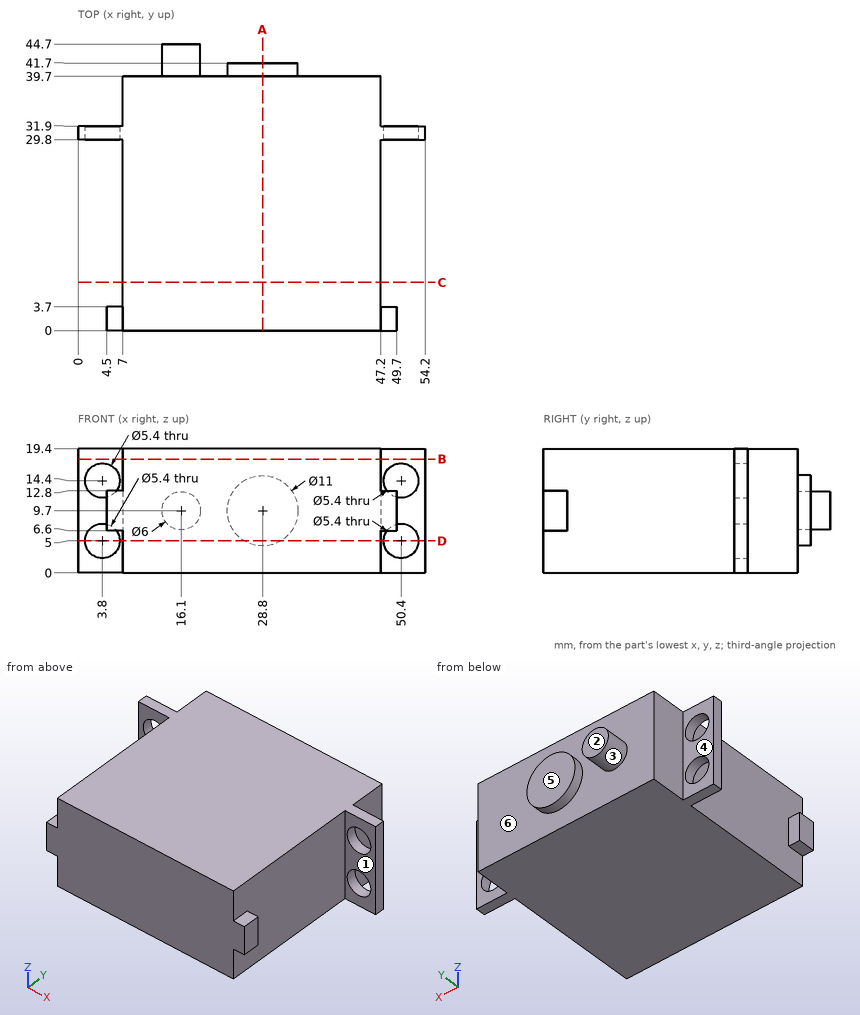
Design review of the part shown in the three views and the two pictorial views. Dimensions are in mm from the part's minimum x, y and z. A direction names the side the tool comes from. Coordinates: 2 decimals unless noted, no trailing zeros. Loops run counter-clockwise (first coordinate to the right, second up) from the corner with the lowest first, then second, coordinate; pieces in that order, holes last. Notation, with made-up numbers: M 3,23.5 L 9,23.5 A28 cw 9,43.5 Z; hole C 65,81 d9. An arc over 180 degrees is marked long. Put each result on its own line as item: value. Start each with the question number.
Q1. Clearance check with flat-ended pins moving along their axes: pin 1 (3 mm diameter, centred on x = 50.4, z = 5, fed in from +Y); pin 2 (2.5 mm diameter, centred on y = 36, z = 11, fed in from +X); pin 3 (1.2 mm diameter, centred on x = 48.5, y = 2.5, fed in from +Z); pin 4 (1.1 mm diameter, centred on y = 2.5, z = 10.5, fed in from -X). State where each tip first meets the part, or that it passes through.
Q2. For the marked faces 4, 5 and 6, list the 3-axis set-ups (+Z, -Z, +X, -X, +Y, -Y) from which the entire face can be reached by the end or side of a thin tool; tool diameter is ignored.
Q3. Add section D-D (z = 5). Write out the cut boundary in (x, y), and give its area (3 significant figures).
Q4. Add section C-C (y = 7.5). Write out the cut boundary in (x, z).
Q5. Add section A-A (x = 28.8). Write out the cut boundary in (y, z).
Q6. The part is to be moulded in two halves that separate along Y. For the marked faces 1, 2 and 3, say which applies: +Y half, -Y half, draft (parallel to the pull), parting line (faces both ways), or undercut.
Q7. Add section B-B (z = 17.75). Write out the cut boundary in (x, y), and give its area (3 significant figures).
Q8. Wall thickness on line 1 (Z direction, x = 50.4, y = 31.45); line 2 (X direction, y = 19.5, z = 16.5); line 3 (Y direction, x = 22.5, z = 16.75): over which ranges is each line inside the solid? List them lowest first.
Answers:
1. pin 1: passes through
1. pin 2: stops at x = 47.2
1. pin 3: stops at z = 12.8
1. pin 4: stops at x = 4.5
2. face 4: +Z, -Z, -X, +Y
2. face 5: +Z, -Z, +X, +Y
2. face 6: +Y
3. outline: M 0,29.8 L 1.1,29.8 L 1.1,31.9 L 0,31.9 Z; M 6.5,29.8 L 7,29.8 L 7,0 L 47.2,0 L 47.2,29.8 L 47.7,29.8 L 47.7,31.9 L 47.2,31.9 L 47.2,39.7 L 31.66,39.7 L 31.66,41.7 L 25.94,41.7 L 25.94,39.7 L 7,39.7 L 7,31.9 L 6.5,31.9 Z; M 53.1,29.8 L 54.2,29.8 L 54.2,31.9 L 53.1,31.9 Z
3. area: 1,610 mm^2
4. outline: M 7,0 L 47.2,0 L 47.2,19.4 L 7,19.4 Z
5. outline: M 0,0 L 39.7,0 L 39.7,4.2 L 41.7,4.2 L 41.7,15.2 L 39.7,15.2 L 39.7,19.4 L 0,19.4 Z
6. face 1: undercut
6. face 2: +Y half
6. face 3: draft
7. outline: M 0,29.8 L 7,29.8 L 7,0 L 47.2,0 L 47.2,29.8 L 54.2,29.8 L 54.2,31.9 L 47.2,31.9 L 47.2,39.7 L 7,39.7 L 7,31.9 L 0,31.9 Z
7. area: 1,630 mm^2
8. line 1: z = 0 to 2.3, 7.7 to 11.7, 17.1 to 19.4
8. line 2: x = 7 to 47.2
8. line 3: y = 0 to 39.7
